Source: CAD feature listing. Evaluate the final solid. Frame: model axes, mm. A direction names the side the tool comes from. Give positions to 0.01 mm unless a question says otherwise; leave off trailing zeros. Order: outer loops, then holes, each group sorted by start corner. A loop starts at its lowest first (then second) coordinate and runs counter-clockwise, first axis right, second up.
from build123d import *

# Parameters (mm, degrees)
ESTRUSIONE_ESTRUSIONE1_DEPTH = 20
SCHIZZO3_R                   = 6
TAGLIO_ESTRUSIONE1_DEPTH     = 26.699370322
SCHIZZO4_W                   = 1.5
SCHIZZO4_H                   = 14.04705955
TAGLIO_ESTRUSIONE2_DEPTH     = 26.699370322
SCHIZZO5_R                   = 15
TAGLIO_ESTRUSIONE3_DEPTH     = 1.5
TAGLIO_ESTRUSIONE4_REACH     = 30.403
SCHIZZO6_R                   = 4.046600507
SMUSSO2_SIZE                 = 0.5
SMUSSO3_SIZE                 = 0.5


with BuildPart() as part:
    # Schizzo2 → Estrusione-Estrusione1 (new body)
    with BuildSketch(Plane.XY):
        with BuildLine():
            Line((8, -13.983665425), (-8, -13.983665425))
            Line((-8, -13.983665425), (-8, 6.016334575))
            ThreePointArc((-8, 6.016334575), (0, 14.016334575), (8, 6.016334575))
            Line((8, 6.016334575), (8, -13.983665425))
        make_face()
    extrude(amount=-ESTRUSIONE_ESTRUSIONE1_DEPTH)

    # Schizzo3 → Taglio-Estrusione1 (cut, through all)
    with BuildSketch(Plane.XY):
        with Locations((0, 6.016334575)):
            Circle(SCHIZZO3_R)
    extrude(amount=-TAGLIO_ESTRUSIONE1_DEPTH, mode=Mode.SUBTRACT)

    # Schizzo4 → Taglio-Estrusione2 (cut, through all)
    with BuildSketch(Plane.XY):
        with Locations((0, -6.96013565)):
            Rectangle(SCHIZZO4_W, SCHIZZO4_H)
    extrude(amount=-TAGLIO_ESTRUSIONE2_DEPTH, mode=Mode.SUBTRACT)

    # Schizzo5 → Taglio-Estrusione3 (cut)
    with BuildSketch(Plane(origin=(8, 0, 0), x_dir=(0, 0, -1), z_dir=(1, 0, 0))):
        with Locations((10, -13.983665425)):
            Circle(SCHIZZO5_R)
    extrude(amount=-TAGLIO_ESTRUSIONE3_DEPTH, mode=Mode.SUBTRACT)

    # Schizzo6 → Taglio-Estrusione4 (cut, up to next)
    with BuildSketch(Plane(origin=(6.5, 0, 0), x_dir=(0, 0, -1), z_dir=(1, 0, 0)), mode=Mode.PRIVATE) as taglio_estrusione4_sk1:
        with Locations((10, -7.483665425)):
            Circle(SCHIZZO6_R)
    taglio_estrusione4_tool1 = extrude(taglio_estrusione4_sk1.sketch, amount=-TAGLIO_ESTRUSIONE4_REACH, mode=Mode.PRIVATE) & part.part
    add(taglio_estrusione4_tool1.solids().sort_by_distance((6.5, -7.483665, -10))[0], mode=Mode.SUBTRACT)

    # Smusso2
    smusso2_edges = [part.edges().sort_by_distance(p)[0] for p in [
        (0, 12.016334575, 0),
    ]]
    chamfer(smusso2_edges, length=SMUSSO2_SIZE)

    # Smusso3
    smusso3_edges = [part.edges().sort_by_distance(p)[0] for p in [
        (0, 12.016334575, -20),
    ]]
    chamfer(smusso3_edges, length=SMUSSO3_SIZE)


solid = part.part
1) Section query C-C on y = -4. Output: boundary loops of the cut face in (x, z), and give its area (3 significant figures).
Checks:
outline: (-8, -20) - (-0.75, -20) - (-0.75, 0) - (-8, 0) - close; (0.75, -20) - (6.5, -20) - (6.5, -12.06) - (0.75, -12.06) - close; (0.75, -7.94) - (6.5, -7.94) - (6.5, 0) - (0.75, 0) - close
area: 236 mm2
2) Reachability of faces 4 (the face through (-0.75, -7, -10)), 5 (the face through (6.5, -3, -10)), 6 (the face through (3.67, -6.27, -13.86)) from +Z, -Z, +X, -X, +Y, -Y: full face, straight path, thin tool, end or side. Return the list, or none.
Checks:
face 4: +Z, -Z, -Y
face 5: +X, -Y
face 6: +X
3) First-contact query: pin 1 Ø5 at (x, z) = (3.5, -3) entering from +Y; pin 2 Ø12 at (y, z) = (-3, -5) entering from +X; pin 3 Ø2 at (y, z) = (9.5, -5) entering from -X; pin 4 Ø7 at (x, y) = (0, 6.02) entering from -Z. Flat tips, straight axial feed; report the tip coordinate or a pass-through.
Checks:
pin 1: stops at y = 13.95
pin 2: stops at x = 8
pin 3: stops at x = -7.6
pin 4: passes through
4) Ray query, L1, parallel to X at y = -0.75, z = -13.75; L2, parallel to Y at x = 3, z = -7. Return the intervals inside material, ascending.
Checks:
L1: x = -8 to -0.75, 0.75 to 6.5
L2: y = -13.98 to -10.2, -4.77 to 0.82, 11.21 to 13.43
5) Section query D-D on x = 2. State how many separate pieces and enclosed holes the cut face has, and give its area (3 significant figures).
Checks:
separate pieces: 2
enclosed holes: 1
area: 277 mm2
6) Section query B-B on x = 0. Output: boundary loops of the cut face in (y, z).
Checks:
outline: (12.02, -19.5) - (12.52, -20) - (14.02, -20) - (14.02, 0) - (12.52, 0) - (12.02, -0.5) - close
7) Section query A-A on z = -10. Output: boundary loops of the cut face in (x, y), and give its area (3 significant figures).
Checks:
outline: (-8, -13.98) - (-0.75, -13.98) - (-0.75, 0.06) arc R6 cw (long way) to (0.75, 0.06) - (0.75, -3.44) - (6.5, -3.44) - (6.5, 1.02) - (8, 1.02) - (8, 6.02) arc R8 ccw to (-8, 6.02) - close; (0.75, -13.98) - (6.5, -13.98) - (6.5, -11.53) - (0.75, -11.53) - close
area: 217 mm2
8) Pull-direction query (Y, two-part tool) for faces 1 (the face through (-0.176, 14.014, -9.86)), 2 (the face through (0.26, 12.15, -19.64)), 3 (the face through (-2, -3, 0)); classes: +Y half, -Y half, draft (parallel to the pull), parting line (faces both ways), or undercut.
Checks:
face 1: +Y half
face 2: undercut
face 3: draft
